Design review of the part built by this model. Coordinates are the model's own, in mm. A direction names the side the tool comes from. Coordinates: 2 decimals unless noted, no trailing zeros. Order: outer loops, then holes, each group sorted by start corner. A loop starts at its lowest first (then second) coordinate and runs counter-clockwise, first axis right, second up. Notation, with made-up numbers: (39, -33.5) -> (43, -33.5) arc R21 ccw to (43, -14.5) -> close; hole circle Ø5 at (13, 74). An arc over 180 degrees is marked (long way). Write item = value, one per line.
```python
from build123d import *

# Parameters (mm, degrees)
F0_R     = 6.425
F1_DEPTH = 12
F2_R     = 1.5
F3_DEPTH = 12.5
F5_DEPTH = 1.75
F6_W     = 3.5
F6_H     = 0.3499913151
F6_W_2   = 2.4
F6_H_2   = 1.6
F6_H_3   = 3
F6_H_4   = 1.8378814235
F7_DEPTH = 12.5
F8_R     = 1.25
F9_DEPTH = 4.5


with BuildPart() as f1:
    # F0 (on Top) → F1 (new body)
    with BuildSketch(Plane.XY):
        Circle(F0_R)
    extrude(amount=-F1_DEPTH)

    # F2 (on Front) → F3 (cut, symmetric)
    with BuildSketch(Plane.XZ):
        with Locations((0, -8.6621185765)):
            Circle(F2_R)
    extrude(amount=F3_DEPTH, both=True, mode=Mode.SUBTRACT)

    # F4 (on Front) → F5 (cut, symmetric)
    with BuildSketch(Plane.XZ):
        with BuildLine():
            Line((6.425, -12), (2.7726078369, -6.7377301586))
            ThreePointArc((2.7726078369, -6.7377301586), (0, -5.2871185765), (-2.7726078369, -6.7377301586))
            Line((-2.7726078369, -6.7377301586), (-6.425, -12))
            Line((-6.425, -12), (6.425, -12))
        make_face()
    extrude(amount=F5_DEPTH, both=True, mode=Mode.SUBTRACT)

    # F6 (on Right) → F7 (cut, symmetric)
    with BuildSketch(Plane.YZ):
        with Locations((0, -11.8250043425)):
            Rectangle(F6_W, F6_H)
        with Locations((-5.225, -6.3621185765)):
            Rectangle(F6_W_2, F6_H_2)
        with Locations((-5.225, -8.6621185765)):
            Rectangle(F6_W_2, F6_H_3)
        with Locations((-5.225, -11.0810592882)):
            Rectangle(F6_W_2, F6_H_4)
    extrude(amount=F7_DEPTH, both=True, mode=Mode.SUBTRACT)

    # F8 (on face) → F9 (join)
    with BuildSketch(Plane.XY):
        Circle(F8_R)
    extrude(amount=F9_DEPTH)


solid = f1.part
```
(1) We need section B-B (y = 0). Write out the cut boundary in (x, z) (3 decimals), and give its area (3 significant figures).
Report:
outline = (-6.425, -11.65) -> (-6.182, -11.65) -> (-2.773, -6.738) arc R3.375 cw to (2.773, -6.738) -> (6.182, -11.65) -> (6.425, -11.65) -> (6.425, 0) -> (1.25, 0) -> (1.25, 4.5) -> (-1.25, 4.5) -> (-1.25, 0) -> (-6.425, 0) -> close
area = 111 mm²
(2) Insertion check: pin 1 (1 mm diameter, centred on x = -4, z = -10, fed in from -Y) (3 decimals); pin 2 (1.8 mm diameter, centred on x = 0, z = -8.66, fed in from -Y); pin 3 (1.9 mm diameter, centred on x = 1, y = -6, fed in from -Z); pin 4 (3.5 mm diameter, centred on x = 1.5, z = -9, fed in from +Y). Each pin has a flat end and moves straight along its axis. Give the tip position at first contact, or say it passes through.
Report:
pin_1 = -4.025
pin_2 = through
pin_3 = -5.56
pin_4 = 6.42
(3) For faces 5 (the cylindrical face through (0.046, -0.024, -5.287)), 6 (the flat face through (0, 4, -12)), 7 (the flat face through (1, -4.025, -10)), list the 3-axis set-ups (+Z, -Z, +X, -X, +Y, -Y) from which the entire face can be reached by the end or side of a thin tool; tool diameter is ignored.
Report:
face_5 = -Z
face_6 = -Z, +X, -X, +Y, -Y
face_7 = -Z, +X, -X, -Y
(4) We need section A-A (x = 0). Write out the cut boundary in (y, z) (3 decimals).
Report:
outline = (-6.425, -5.562) -> (-4.025, -5.562) -> (-4.025, -7.162) -> (-1.75, -7.162) -> (-1.75, -5.287) -> (1.75, -5.287) -> (1.75, -7.162) -> (6.425, -7.162) -> (6.425, 0) -> (1.25, 0) -> (1.25, 4.5) -> (-1.25, 4.5) -> (-1.25, 0) -> (-6.425, 0) -> close; (-4.025, -12) -> (-1.75, -12) -> (-1.75, -10.162) -> (-4.025, -10.162) -> close; (1.75, -12) -> (6.425, -12) -> (6.425, -10.162) -> (1.75, -10.162) -> close
(5) The part is to be moulded in two halves that separate along Z. For faces 1 (the cylindrical face through (-0.27, -1.22, 2.22)), 2 (the flat face through (0, -5, -5.562)), 3 (the cylindrical face through (-0.325, -2.903, -10.126)), 4 (the flat face through (0, 0, 4.5)), say which applies: released by +Z, released by -Z, zero draft, split by the parting line, or undercut.
Report:
face_1 = zero draft
face_2 = released by -Z
face_3 = undercut
face_4 = released by +Z
(6) We need section C-C (x = 3.5). Write out the cut boundary in (y, z) (3 decimals), and give its area (3 significant figures).
Report:
outline = (-5.388, -5.562) -> (-4.025, -5.562) -> (-4.025, -12) -> (-1.75, -12) -> (-1.75, -7.786) -> (1.75, -7.786) -> (1.75, -12) -> (5.388, -12) -> (5.388, 0) -> (-5.388, 0) -> close
area = 106 mm²
(7) We need section D-D (y = 5.75). Write out the cut boundary in (x, z).
Report:
outline = (-2.87, -12) -> (2.87, -12) -> (2.87, 0) -> (-2.87, 0) -> close; hole circle Ø3 at (0, -8.66)
(8) For L1, parallel to Z at x = 0, y = -3; L2, parallel to Z at x = 4.5, y = 3.5; L3, parallel to Z at x = -2.5, y = -5, list the stretches that pass through material, from the lowest coordinate up.
Report:
L1 = -12 to -10.16, -7.16 to 0
L2 = -12 to 0
L3 = -5.56 to 0
